CAD build for the part. Positions are in the model's coordinates, mm. A direction names the side the tool comes from. Give positions to 0.01 mm unless a question says otherwise; leave off trailing zeros. Order: outer loops, then holes, each group sorted by start corner. A loop starts at its lowest first (then second) coordinate and runs counter-clockwise, first axis right, second up.
from build123d import *

# Parameters (mm, degrees)
EXTRUDE_2_DEPTH     = 3
SKETCH_4_R          = 2.25
SKETCH_4_R_2        = 2.5
CUT_EXTRUDE_2_DEPTH = 96.402519291
SKETCH_6_R          = 3.5
CUT_EXTRUDE_3_DEPTH = 96.402519291
SKETCH_7_R          = 3.5
CUT_EXTRUDE_4_DEPTH = 96.402519291
CUT_EXTRUDE_5_DEPTH = 96.402519291
EXTRUDE_4_DEPTH     = 15


with BuildPart() as part:
    # 草图2 → 凸台-拉伸2 (new body)
    with BuildSketch(Plane(origin=(0, 0, 0), x_dir=(1, 0, 0), z_dir=(0, 1, 0))):
        with BuildLine():
            Line((-58.569449541, 23.337085947), (32.740581269, -53.879999426))
            ThreePointArc((32.740581269, -53.879999426), (53.033008589, -53.033008589), (53.879999426, -32.740581269))
            Line((53.879999426, -32.740581269), (-23.337085947, 58.569449541))
            ThreePointArc((-23.337085947, 58.569449541), (-60.104076401, 60.104076401), (-58.569449541, 23.337085947))
        make_face()
    extrude(amount=EXTRUDE_2_DEPTH)

    # 草图4 → 切除-拉伸2 (cut, through all)
    with BuildSketch(Plane(origin=(0, 3, 0), x_dir=(1, 0, 0), z_dir=(0, 1, 0))):
        with Locations(Location((-42.426406871, 42.426406871, 0), (0, 0, 270))):
            Circle(SKETCH_4_R)
        with Locations(Location((42.426406871, -42.426406871, 0), (0, 0, 270))):
            Circle(SKETCH_4_R_2)
    extrude(amount=-CUT_EXTRUDE_2_DEPTH, mode=Mode.SUBTRACT)

    # 草图6 → 切除-拉伸3 (cut, through all)
    with BuildSketch(Plane(origin=(0, 3, 0), x_dir=(1, 0, 0), z_dir=(0, 1, 0))):
        with Locations(Location((-42.426406871, 42.426406871, 0), (0, 0, 270))):
            Circle(SKETCH_6_R)
    extrude(amount=-CUT_EXTRUDE_3_DEPTH, mode=Mode.SUBTRACT)

    # 草图7 → 切除-拉伸4 (cut, through all)
    with BuildSketch(Plane(origin=(0, 3, 0), x_dir=(1, 0, 0), z_dir=(0, 1, 0))):
        with Locations(Location((42.426406871, -42.426406871, 0), (0, 0, 270))):
            Circle(SKETCH_7_R)
    extrude(amount=-CUT_EXTRUDE_4_DEPTH, mode=Mode.SUBTRACT)

    # 草图8 → 切除-拉伸5 (cut, through all)
    with BuildSketch(Plane(origin=(0, 3, 0), x_dir=(1, 0, 0), z_dir=(0, 1, 0))):
        Polygon((33.626672858, -22.564710472), (-15.702999665, 25.870376375), (-26.891422763, 12.98046534), (25.218843822, -32.251166492), align=None)
    extrude(amount=-CUT_EXTRUDE_5_DEPTH, mode=Mode.SUBTRACT)

    # 草图9 → 凸台-拉伸4 (add)
    with BuildSketch(Plane(origin=(0, 3, 0), x_dir=(1, 0, 0), z_dir=(0, 1, 0))):
        with BuildLine():
            ThreePointArc((-17.960284018, 47.565359346), (-19.96440182, 53.401757848), (-23.337085947, 58.569449541))
            ThreePointArc((-23.337085947, 58.569449541), (-60.104076401, 60.104076401), (-58.569449541, 23.337085947))
            ThreePointArc((-58.569449541, 23.337085947), (-53.401757848, 19.96440182), (-47.565359346, 17.960284018))
            Line((-47.565359346, 17.960284018), (-56.632284421, 25.627804458))
            ThreePointArc((-56.632284421, 25.627804458), (-57.982756057, 57.982756057), (-25.627804458, 56.632284421))
            Line((-25.627804458, 56.632284421), (-17.960284018, 47.565359346))
        make_face()
        with BuildLine():
            Line((53.879999426, -32.740581269), (-23.337085947, 58.569449541))
            ThreePointArc((-23.337085947, 58.569449541), (-19.96440182, 53.401757848), (-17.960284018, 47.565359346))
            Line((-17.960284018, 47.565359346), (45.777785554, -27.805590857))
            ThreePointArc((45.777785554, -27.805590857), (50.229311839, -29.615681908), (53.879999426, -32.740581269))
        make_face()
        with BuildLine():
            ThreePointArc((-47.565359346, 17.960284018), (-53.401757848, 19.96440182), (-58.569449541, 23.337085947))
            Line((-58.569449541, 23.337085947), (32.740581269, -53.879999426))
            ThreePointArc((32.740581269, -53.879999426), (29.615681908, -50.229311839), (27.805590857, -45.777785554))
            Line((27.805590857, -45.777785554), (-47.565359346, 17.960284018))
        make_face()
        with BuildLine():
            ThreePointArc((57.426406871, -42.426406871), (56.511929373, -37.26907657), (53.879999426, -32.740581269))
            ThreePointArc((53.879999426, -32.740581269), (50.229311839, -29.615681908), (45.777785554, -27.805590857))
            Line((45.777785554, -27.805590857), (51.589280915, -34.67774639))
            ThreePointArc((51.589280915, -34.67774639), (53.694824873, -38.30054263), (54.426406871, -42.426406871))
            ThreePointArc((54.426406871, -42.426406871), (47.47695507, -53.311808237), (34.67774639, -51.589280915))
            Line((34.67774639, -51.589280915), (27.805590857, -45.777785554))
            ThreePointArc((27.805590857, -45.777785554), (29.615681908, -50.229311839), (32.740581269, -53.879999426))
            ThreePointArc((32.740581269, -53.879999426), (48.73959212, -56.033158578), (57.426406871, -42.426406871))
        make_face()
    extrude(amount=EXTRUDE_4_DEPTH)


solid = part.part
1. 3-axis set-ups, long thin cutter, end or side, ignore diameter. For faces 1 (the flat face through (-21.219, 1.521, -19.516)), 2 (the flat face through (9, 18, -19)), 3 (the flat face through (-5, 3, -18)): which of +Z, -Z, +X, -X, +Y, -Y reach the whole face in a straight line?
2. Mould opens along X. For faces 4 (the flat face through (-15, 0, -1)), 5 (the cylindrical face through (45.9, 1.5, 42)), 6 (the flat face through (15.81, 8.87, -12.28)), 7 (the flat face through (-1.2, 1.52, 9.32)) say: released by +X, released by -X, zero draft, split by the parting line, or undercut.
3. Saw through at C-C on z = 5.5. Give the cut face in (x, y).
4. Saw through at D-D on z = 48.5. Give the cut face in (x, y).
5. Wall check: line 1 (X direction, y = 8, z = 45); line 2 (Z direction, x = 14, y = 15.75); line 3 (Y direction, x = -56.5, z = -55). Give the ranges that are in metal, low to high.
6. Saw through at B-B on x = -21.5. Give the cut face in (y, z), plus the area to 3 significant figures.
7. Pin check, flat tips, straight feed: P1, Ø2, axis at y = 11.5, z = -10, coming from the +X side; P2, Ø1.5, axis at y = 4, z = 9, coming from the -X side; P3, Ø3, axis at y = 6.5, z = 13, coming from the -X side. Stop position of each tip, or through.
8. Saw through at A-A on y = 6.25. Give the cut face in (x, z).
Reported:
1. face 1: +Y, -Y
1. face 2: +Z, -Z, +X, -X, +Y
1. face 3: +Y
2. face 4: zero draft
2. face 5: undercut
2. face 6: released by +X
2. face 7: undercut
3. outline: (-24.47, 0) - (-5.6, 0) - (-5.6, 3) - (-19.82, 3) - (-19.82, 18) - (-24.47, 18) - close; (16.25, 0) - (30.84, 0) - (30.84, 18) - (26.91, 18) - (26.91, 3) - (16.25, 3) - close
4. outline: (26.38, 0) - (56.14, 0) - (56.14, 18) - (52.78, 18) - (52.78, 3) - (31.02, 3) - (31.02, 18) - (26.38, 18) - close
5. line 1: x = 22.24 to 26.89, 54.15 to 57.2
5. line 2: z = -14.42 to -9.77, 34.1 to 38.03
5. line 3: y = 0 to 3
6. outline: (0, -56.4) - (18, -56.4) - (18, -51.75) - (3, -51.75) - (3, -19.19) - (0, -19.19) - close; (0, -8.3) - (3, -8.3) - (3, 4.08) - (18, 4.08) - (18, 8.01) - (0, 8.01) - close
6. area: 289 mm2
7. P1: stops at x = 18.58
7. P2: stops at x = -21.22
7. P3: stops at x = -17.37
8. outline: (-58.57, -23.34) arc R25 ccw (long way) to (-23.34, -58.57) - (53.88, 32.74) arc R15 ccw to (32.74, 53.88) - close; hole (-56.63, -25.63) arc R22 ccw (long way) to (-25.63, -56.63) - (51.59, 34.68) arc R12 ccw to (34.68, 51.59) - close
